Check sheet for the drawn part. Datum: minimum x, y, z corner. Units: mm. Round coordinates to 2 decimals unless told otherwise and drop trailing zeros.
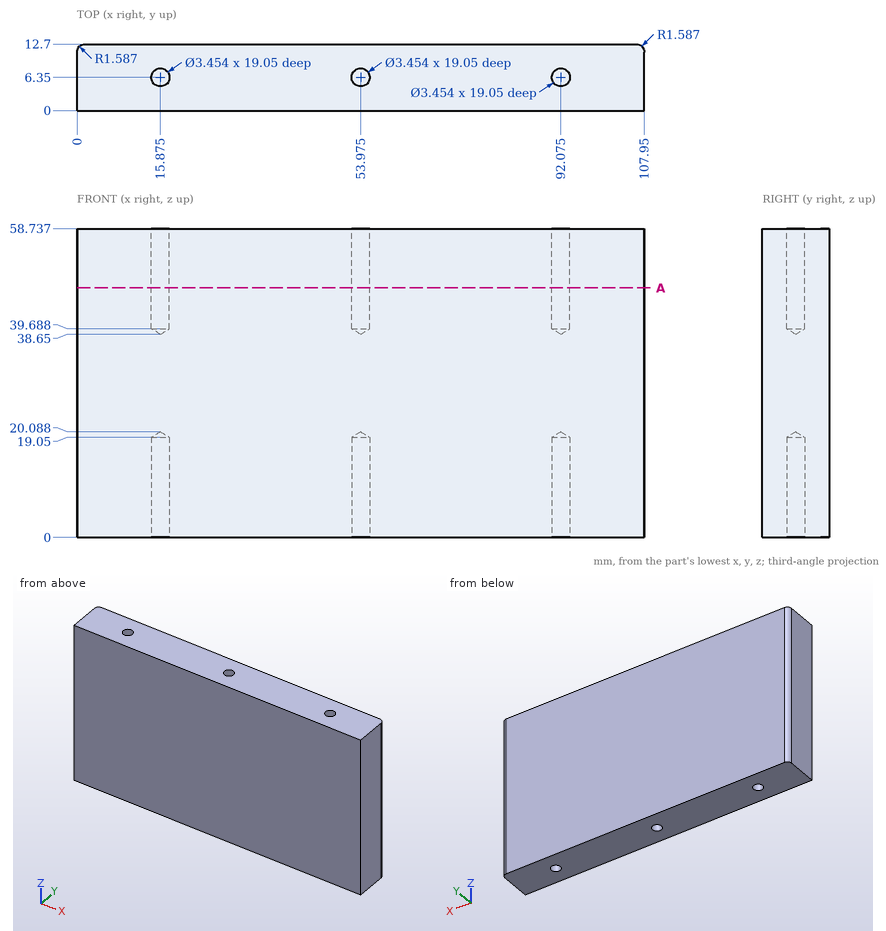
(1) Depth check by flat-ended pin: P1, Ø2, axis at x = 92.075, y = 6.35, coming from the +Z side; P2, Ø3, axis at x = 15.875, y = 6.35, coming from the -Z side; P3, Ø3, axis at x = 53.975, y = 6.35, coming from the +Z side. Enter the tip coordinate at first touch or a pass-through.
Returned:
P1: stops at z = 39.25
P2: stops at z = 19.19
P3: stops at z = 39.55
(2) Sectioned sample at A-A, the plane z = 47.5. Give the number of separate pieces and of enclosed holes in the cut face, and give its area (3 significant figures).
Returned:
separate pieces: 1
enclosed holes: 3
area: 1,340 mm2
(3) Material ranges on line 1 (X direction, y = 6.35, z = 49.5); line 2 (X direction, y = 7.25, z = 48); line 3 (X direction, y = 11.75, z = 6.5) (1 decimal), recorded low to high.
Returned:
line 1: x = 0 to 14.15, 17.6 to 52.25, 55.7 to 90.35, 93.8 to 107.95
line 2: x = 0 to 14.4, 17.35 to 52.5, 55.45 to 90.6, 93.55 to 107.95
line 3: x = 0.1 to 107.8
